CAD build for the part. Positions are in the model's coordinates, mm. Round coordinates to 2 decimals unless told otherwise and drop trailing zeros. Loops run counter-clockwise (first coordinate to the right, second up) from the corner with the lowest first, then second, coordinate; pieces in that order, holes last.
from build123d import *

# Parameters (mm, degrees)
F2_SIZE = 1
F3_R    = 1


with BuildPart() as f1:
    # F0 (on Front) → F1 (revolve)
    with BuildSketch(Plane.XZ):
        with BuildLine():
            Line((-12.5, 22.996796), (-12.5, 0))
            Line((-12.5, 0), (-3, 0))
            Line((-3, 0), (-3, 15))
            Line((-3, 15), (0, 15))
            Line((0, 15), (0, 25.913464))
            ThreePointArc((0, 25.913464), (-6.422136, 25.192857), (-12.5, 22.996796))
        make_face()
    revolve(axis=Axis((0, 0, 20.456732), (0, 0, 1)))

    # F2
    f2_edges = [f1.edges().sort_by_distance(p)[0] for p in [
        (3, 0, 0),
    ]]
    chamfer(f2_edges, length=F2_SIZE)

    # F3
    f3_edges = [f1.edges().sort_by_distance(p)[0] for p in [
        (12.5, 0, 22.996796),
    ]]
    fillet(f3_edges, radius=F3_R)


solid = f1.part
Item 1: Cut at B-B (z = 18.5). List the corners of the cut face in (x, y).
Verdict:
outline: circle Ø25 at (0, 0)
Item 2: Mould opens along X. For faces 1 (the cylindrical face through (3, 0, 8)), 2 (the flat face through (3, -3, 0)), 3 (the cylindrical face through (-11.923, -3.755, 11.029)) say: released by +X, released by -X, zero draft, split by the parting line, or undercut.
Verdict:
face 1: undercut
face 2: zero draft
face 3: split by the parting line
Item 3: Cut at A-A (z = 10.5). List the corners of the cut face in (x, y).
Verdict:
outline: circle Ø25 at (0, 0); hole circle Ø6 at (0, 0)
Item 4: Flat gauge pins, fed straight in: P1, Ø8, axis at y = 5, z = 20, coming from the -X side; P2, Ø2, axis at x = -7.5, z = 3, coming from the +Y side; P3, Ø10, axis at x = 5, y = -1.5, coming from the -Z side; P4, Ø8, axis at x = -7.5, z = 6, coming from the +Y side. Where does each tip first touch, or does it go through?
Verdict:
P1: stops at x = -12.46
P2: stops at y = 10.68
P3: stops at z = 0
P4: stops at y = 12
Item 5: Wall check: L1, parallel to Y at x = 0, z = 11.5; L2, parallel to Z at x = -10, y = -6.5. Give the ranges that are in metal, low to high.
Verdict:
L1: y = -12.5 to -3, 3 to 12.5
L2: z = 0 to 23.28
